The listing builds one solid part. Answer for the finished solid, in the listing's coordinates (mm). A direction names the side the tool comes from. Coordinates: 2 decimals unless noted, no trailing zeros. Order: outer loops, then holes, each group sorted by start corner. A loop starts at its lowest first (then second) coordinate and runs counter-clockwise, first axis right, second up. Notation, with made-up numbers: (-17, -11) -> (-8, -11) arc R18 cw to (-8, 7) -> close; hole circle Ø8 at (9.5, 0). An arc over 180 degrees is marked (long way). Return JSON: item names as keys, results as strings.
from build123d import *

# Parameters (mm, degrees)
BOSS_EXTRUDE1_DEPTH  = 10
BOSS_EXTRUDE3_DEPTH  = 4.5
BOSS_EXTRUDE4_DEPTH  = 8.5
SKETCH5_R            = 11
BOSS_EXTRUDE5_DEPTH  = 2
CUT_EXTRUDE1_REACH   = 39.563
SKETCH6_R            = 1.5
SKETCH7_R            = 5.5
CUT_EXTRUDE2_DEPTH   = 3.5
SKETCH8_R            = 2.5
BOSS_EXTRUDE6_DEPTH  = 3.5
BOSS_EXTRUDE7_DEPTH  = 19.5
SKETCH10_R           = 3.5
CUT_EXTRUDE3_DEPTH   = 3
SKETCH11_W           = 17
SKETCH11_H           = 3
BOSS_EXTRUDE8_DEPTH  = 5
SKETCH12_W           = 16.5
SKETCH12_H           = 6
BOSS_EXTRUDE9_DEPTH  = 7.5
SKETCH13_W           = 15
SKETCH13_H           = 3.5
CUT_EXTRUDE4_DEPTH   = 5.5
CUT_EXTRUDE5_REACH   = 52.135
SKETCH14_W           = 8.5
SKETCH14_H           = 5.5
SKETCH15_W           = 1.5
SKETCH15_H           = 5.5
CUT_EXTRUDE6_DEPTH   = 1.25
SKETCH16_R           = 0.375
BOSS_EXTRUDE10_DEPTH = 5.5


with BuildPart() as part:
    # Sketch1 → Boss-Extrude1 (new body)
    with BuildSketch(Plane(origin=(0, 0, 0), x_dir=(1, 0, 0), z_dir=(0, 1, 0))):
        Polygon((-21, 16.5), (-16.5, 21), (16.5, 21), (21, 16.5), (21, -16.5), (16.5, -21), (-16.5, -21), (-21, -16.5), align=None)
    extrude(amount=BOSS_EXTRUDE1_DEPTH)

    # Sketch2 → Boss-Extrude3 (add)
    with BuildSketch(Plane(origin=(0, 10, 0), x_dir=(1, 0, 0), z_dir=(0, 1, 0))):
        with BuildLine():
            Line((-15.318019485, 19.681980515), (-19.681980515, 15.318019485))
            ThreePointArc((-19.681980515, 15.318019485), (-20.657457896, 13.858114415), (-21, 12.136038969))
            Line((-21, 12.136038969), (-21, -12.136038969))
            ThreePointArc((-21, -12.136038969), (-20.657457896, -13.858114415), (-19.681980515, -15.318019485))
            Line((-19.681980515, -15.318019485), (-15.318019485, -19.681980515))
            ThreePointArc((-15.318019485, -19.681980515), (-13.858114415, -20.657457896), (-12.136038969, -21))
            Line((-12.136038969, -21), (12.136038969, -21))
            ThreePointArc((12.136038969, -21), (13.858114415, -20.657457896), (15.318019485, -19.681980515))
            Line((15.318019485, -19.681980515), (19.681980515, -15.318019485))
            ThreePointArc((19.681980515, -15.318019485), (20.657457896, -13.858114415), (21, -12.136038969))
            Line((21, -12.136038969), (21, 12.136038969))
            ThreePointArc((21, 12.136038969), (20.657457896, 13.858114415), (19.681980515, 15.318019485))
            Line((19.681980515, 15.318019485), (15.318019485, 19.681980515))
            ThreePointArc((15.318019485, 19.681980515), (13.858114415, 20.657457896), (12.136038969, 21))
            Line((12.136038969, 21), (-12.136038969, 21))
            ThreePointArc((-12.136038969, 21), (-13.858114415, 20.657457896), (-15.318019485, 19.681980515))
        make_face()
    extrude(amount=BOSS_EXTRUDE3_DEPTH)

    # Sketch4 → Boss-Extrude4 (add)
    with BuildSketch(Plane(origin=(0, 14.5, 0), x_dir=(1, 0, 0), z_dir=(0, 1, 0))):
        Polygon((-16.5, 21), (-21, 16.5), (-21, -16.5), (-16.5, -21), (16.5, -21), (21, -16.5), (21, 16.5), (16.5, 21), align=None)
    extrude(amount=BOSS_EXTRUDE4_DEPTH)

    # Sketch5 → Boss-Extrude5 (add)
    with BuildSketch(Plane(origin=(0, 23, 0), x_dir=(1, 0, 0), z_dir=(0, 1, 0))):
        with Locations(Location((0, 0, 0), (0, 0, 270))):
            Circle(SKETCH5_R)
    extrude(amount=BOSS_EXTRUDE5_DEPTH)

    # Sketch6 → Cut-Extrude1 (cut, up to next)
    with BuildSketch(Plane(origin=(0, 23, 0), x_dir=(1, 0, 0), z_dir=(0, 1, 0)), mode=Mode.PRIVATE) as cut_extrude1_sk1:
        with Locations(Location((-15.5, 15.5, 0), (0, 0, 270))):
            Circle(SKETCH6_R)
    cut_extrude1_tool1 = extrude(cut_extrude1_sk1.sketch, amount=-CUT_EXTRUDE1_REACH, mode=Mode.PRIVATE) & part.part
    # Sketch6 → Cut-Extrude1 (cut, up to next)
    with BuildSketch(Plane(origin=(0, 23, 0), x_dir=(1, 0, 0), z_dir=(0, 1, 0)), mode=Mode.PRIVATE) as cut_extrude1_sk2:
        with Locations(Location((15.5, 15.5, 0), (0, 0, 270))):
            Circle(SKETCH6_R)
    cut_extrude1_tool2 = extrude(cut_extrude1_sk2.sketch, amount=-CUT_EXTRUDE1_REACH, mode=Mode.PRIVATE) & part.part
    # Sketch6 → Cut-Extrude1 (cut, up to next)
    with BuildSketch(Plane(origin=(0, 23, 0), x_dir=(1, 0, 0), z_dir=(0, 1, 0)), mode=Mode.PRIVATE) as cut_extrude1_sk3:
        with Locations(Location((15.5, -15.5, 0), (0, 0, 270))):
            Circle(SKETCH6_R)
    cut_extrude1_tool3 = extrude(cut_extrude1_sk3.sketch, amount=-CUT_EXTRUDE1_REACH, mode=Mode.PRIVATE) & part.part
    # Sketch6 → Cut-Extrude1 (cut, up to next)
    with BuildSketch(Plane(origin=(0, 23, 0), x_dir=(1, 0, 0), z_dir=(0, 1, 0)), mode=Mode.PRIVATE) as cut_extrude1_sk4:
        with Locations(Location((-15.5, -15.5, 0), (0, 0, 270))):
            Circle(SKETCH6_R)
    cut_extrude1_tool4 = extrude(cut_extrude1_sk4.sketch, amount=-CUT_EXTRUDE1_REACH, mode=Mode.PRIVATE) & part.part
    add(cut_extrude1_tool1.solids().sort_by_distance((-15.5, 23, -15.5))[0], mode=Mode.SUBTRACT)
    add(cut_extrude1_tool2.solids().sort_by_distance((15.5, 23, -15.5))[0], mode=Mode.SUBTRACT)
    add(cut_extrude1_tool3.solids().sort_by_distance((15.5, 23, 15.5))[0], mode=Mode.SUBTRACT)
    add(cut_extrude1_tool4.solids().sort_by_distance((-15.5, 23, 15.5))[0], mode=Mode.SUBTRACT)

    # Sketch7 → Cut-Extrude2 (cut)
    with BuildSketch(Plane(origin=(0, 25, 0), x_dir=(1, 0, 0), z_dir=(0, 1, 0))):
        with Locations(Location((0, 0, 0), (0, 0, 270))):
            Circle(SKETCH7_R)
    extrude(amount=-CUT_EXTRUDE2_DEPTH, mode=Mode.SUBTRACT)

    # Sketch8 → Boss-Extrude6 (add)
    with BuildSketch(Plane(origin=(0, 21.5, 0), x_dir=(1, 0, 0), z_dir=(0, 1, 0))):
        with Locations(Location((0, 0, 0), (0, 0, 270))):
            Circle(SKETCH8_R)
    extrude(amount=BOSS_EXTRUDE6_DEPTH)

    # Sketch9 → Boss-Extrude7 (add)
    with BuildSketch(Plane(origin=(0, 25, 0), x_dir=(1, 0, 0), z_dir=(0, 1, 0))):
        with BuildLine():
            Line((-1.5, 2), (1.5, 2))
            ThreePointArc((1.5, 2), (0, -2.5), (-1.5, 2))
        make_face()
    extrude(amount=BOSS_EXTRUDE7_DEPTH)

    # Sketch10 → Cut-Extrude3 (cut)
    with BuildSketch(Plane.XZ):
        with Locations(Location((-15.5, 15.5, 0), (0, 0, 270))):
            Circle(SKETCH10_R)
        with Locations(Location((15.5, 15.5, 0), (0, 0, 270))):
            Circle(SKETCH10_R)
        with Locations(Location((15.5, -15.5, 0), (0, 0, 270))):
            Circle(SKETCH10_R)
        with Locations(Location((-15.5, -15.5, 0), (0, 0, 270))):
            Circle(SKETCH10_R)
    extrude(amount=-CUT_EXTRUDE3_DEPTH, mode=Mode.SUBTRACT)

    # Sketch11 → Boss-Extrude8 (add)
    with BuildSketch(Plane.XY.offset(21)):
        with Locations((0, 1.5)):
            Rectangle(SKETCH11_W, SKETCH11_H)
    extrude(amount=BOSS_EXTRUDE8_DEPTH)

    # Sketch12 → Boss-Extrude9 (add)
    with BuildSketch(Plane.XY.offset(21)):
        with Locations((0, 6)):
            Rectangle(SKETCH12_W, SKETCH12_H)
    extrude(amount=BOSS_EXTRUDE9_DEPTH)

    # Sketch13 → Cut-Extrude4 (cut)
    with BuildSketch(Plane.XY.offset(28.5)):
        with Locations((0, 6)):
            Rectangle(SKETCH13_W, SKETCH13_H)
    extrude(amount=-CUT_EXTRUDE4_DEPTH, mode=Mode.SUBTRACT)

    # Sketch14 → Cut-Extrude5 (cut, up to next)
    with BuildSketch(Plane(origin=(0, 9, 0), x_dir=(1, 0, 0), z_dir=(0, 1, 0)), mode=Mode.PRIVATE) as cut_extrude5_sk1:
        with Locations((0, -25.75)):
            Rectangle(SKETCH14_W, SKETCH14_H)
    cut_extrude5_tool1 = extrude(cut_extrude5_sk1.sketch, amount=-CUT_EXTRUDE5_REACH, mode=Mode.PRIVATE) & part.part
    add(cut_extrude5_tool1.solids().sort_by_distance((0, 9, 25.75))[0], mode=Mode.SUBTRACT)

    # Sketch15 → Cut-Extrude6 (cut)
    with BuildSketch(Plane(origin=(0, 9, 0), x_dir=(1, 0, 0), z_dir=(0, 1, 0))):
        with Locations((-6.5, -23.75)):
            Rectangle(SKETCH15_W, SKETCH15_H)
        with Locations((6.5, -23.75)):
            Rectangle(SKETCH15_W, SKETCH15_H)
    extrude(amount=-CUT_EXTRUDE6_DEPTH, mode=Mode.SUBTRACT)

    # Sketch16 → Boss-Extrude10 (add)
    with BuildSketch(Plane.XY.offset(23)):
        with Locations(Location((-1.27, 6.25, 0), (0, 0, 180))):
            Circle(SKETCH16_R)
        with Locations(Location((1.27, 6.25, 0), (0, 0, 180))):
            Circle(SKETCH16_R)
        with Locations(Location((-3.81, 6.25, 0), (0, 0, 180))):
            Circle(SKETCH16_R)
        with Locations(Location((-6.35, 6.25, 0), (0, 0, 180))):
            Circle(SKETCH16_R)
        with Locations(Location((3.81, 6.25, 0), (0, 0, 180))):
            Circle(SKETCH16_R)
        with Locations(Location((6.35, 6.25, 0), (0, 0, 180))):
            Circle(SKETCH16_R)
    extrude(amount=BOSS_EXTRUDE10_DEPTH)


solid = part.part
1. Each of these flat-tipped pins is pushed along its axis until it touches: pin 1 Ø5.5 at (x, z) = (-15.5, -15.5) entering from -Y; pin 2 Ø8 at (x, z) = (3, 26.5) entering from +Y; pin 3 Ø4 at (x, y) = (-9, 26.5) entering from -Z. Where does it stop, or does it pass through?
Answer block:
{"pin 1": "stops at y = 3", "pin 2": "stops at y = 9", "pin 3": "stops at z = -7.88"}
2. The part is cut by section A-A on z = 0. Give the vertices of the cut face in (x, y), and give its area (3 significant figures).
Answer block:
{"outline": "(-21, 0) -> (21, 0) -> (21, 23) -> (11, 23) -> (11, 25) -> (5.5, 25) -> (5.5, 21.5) -> (2.5, 21.5) -> (2.5, 44.5) -> (-2.5, 44.5) -> (-2.5, 21.5) -> (-5.5, 21.5) -> (-5.5, 25) -> (-11, 25) -> (-11, 23) -> (-21, 23) -> close", "area": "1,090 mm2"}
3. Determine the mould class of faces 1 (the face through (0, 7, 23)), 2 (the face through (14, 3, 14.8)), 3 (the face through (20.667, 12.218, -13.835)), 4 (the face through (-18, 14.5, 18)) for opening direction Z: pulls with the +Z half, pulls with the -Z half, needs draft (parallel to the pull), parting line crosses it, or undercut.
Answer block:
{"face 1": "pulls with the +Z half", "face 2": "undercut", "face 3": "pulls with the -Z half", "face 4": "needs draft"}
4. The part is cut by section B-B on y = 38.5. Give the vertices of the cut face in (x, z).
Answer block:
{"outline": "(-1.5, -2) -> (1.5, -2) arc R2.5 ccw (long way) to start"}
5. Consider line 1 (X direction, y = 2.15, z = -15.5); line 2 (X direction, y = 7, z = 23.5); line 3 (X direction, y = 18, z = 15.5). Determine where each line is inside the solid, lowest interval first. Write a range as from..to.
Answer block:
{"line 1": "x = -21..-19, -12..12, 19..21", "line 2": "x = -8.25..-7.5, 7.5..8.25", "line 3": "x = -21..-17, -14..14, 17..21"}
6. The part is cut by section C-C on z = 8. Give the vertices of the cut face in (x, y), and give its area (3 significant figures).
Answer block:
{"outline": "(-21, 0) -> (21, 0) -> (21, 23) -> (7.55, 23) -> (7.55, 25) -> (-7.55, 25) -> (-7.55, 23) -> (-21, 23) -> close", "area": "996 mm2"}
7. For faces 5 (the face through (8.5, 1, 23)), 6 (the face through (18, 14.5, -18)), 7 (the face through (20.65, 12.22, 13.88)), 8 (the face through (0, 4.25, 26)), determine the directions among +Z, -Z, +X, -X, +Y, -Y from which every point of the face is accessible in a straight line to the end or side of a thin tool.
Answer block:
{"face 5": "+Z, +X, +Y, -Y", "face 6": "-Z, +X", "face 7": "+Z, +X", "face 8": "+Z"}
